Geometry: final body of the model. Coordinates: model frame, mm. A direction names the side the tool comes from. Round coordinates to 2 decimals unless told otherwise and drop trailing zeros. Order: outer loops, then holes, each group sorted by start corner. A loop starts at its lowest first (then second) coordinate and runs counter-clockwise, first axis right, second up. Notation, with made-up numbers: (-23, 78) - (5, 78) arc R11 cw to (5, 99) - close; hole circle Ø11 at (-5.5, 59.5). An arc over 180 degrees is marked (long way). Put each result on its own line as item: value. Start each with the question number.
(1) Pin query (flat end, axial travel): P1, Ø1, axis at x = 344, z = -137, coming from the +Y side; P2, Ø8, axis at x = -549, z = -4.5, coming from the +Y side; P3, Ø4, axis at y = 0, z = -1803.4, coming from the +X side; P4, Ø1, axis at x = 394.5, y = -102.5, coming from the -Z side. Return the tip coordinate at first contact, or that it passes through.
(2) Access query for faces 1 (the face through (-1, 25.4, -1465)), 2 (the face through (-510.54, -7, -229)), 3 (the face through (684.768, -8.392, -284.552)), 4 (the face through (345.44, -7, -42)), 5 (the face through (-586.74, -7, -228)). Directions: +Z, -Z, +X, -X, +Y, -Y. A direction counts if a zero-diameter tool reaches every point of the face in a straight line with its end or side. Return the directions, or none.
(3) Material intervals for L1, parallel to Z at x = -7.5, y = 0; L2, parallel to Z at x = 6.5, y = 0; L3, parallel to Z at x = 579, y = 201.5, sorted ascending. Write a range as [from, to].
(4) Section D-D (z = -1072.5). Output: boundary loops of the cut face in (x, y).
(5) Section C-C (y = 374). Output: boundary loops of the cut face in (x, z), and give its area (3 significant figures).
(6) Section B-B (x = 0). Output: boundary loops of the cut face in (y, z) (1 decimal).
(7) Section A-A (x = 420). Output: boundary loops of the cut face in (y, z), and give its area (3 significant figures).
(8) Pull-direction query (X, two-part tool) for faces 6 (the face through (-345.44, -7, -48)), 7 (the face through (-2, 36, -1397)), 8 (the face through (242.165, -2.134, -1326.863)), 9 (the face through (-50.8, -1, -996)); classes: released by +X, released by -X, zero draft, split by the parting line, or undercut.
from build123d import *

# Parameters (mm, degrees)
F1_DEPTH      = 599.44
F2_W          = 127
F2_H          = 457.2
F2_R          = 1.5875
F3_DEPTH      = 751.841
F3_DEPTH_BACK = 751.841


with BuildPart() as f1:
    # F0 (on Front) → F1 (new body, symmetric)
    with BuildSketch(Plane.XZ):
        with BuildLine():
            Line((751.84, 203.2), (345.44, 203.2))
            Line((345.44, 203.2), (345.44, -203.2))
            Line((345.44, -203.2), (510.54, -203.2))
            Line((510.54, -203.2), (510.54, -254))
            Line((510.54, -254), (0, -254))
            Line((0, -254), (-510.54, -254))
            Line((-510.54, -254), (-510.54, -203.2))
            Line((-510.54, -203.2), (-345.44, -203.2))
            Line((-345.44, -203.2), (-345.44, 203.2))
            Line((-345.44, 203.2), (-751.84, 203.2))
            Line((-751.84, 203.2), (-751.84, -203.2))
            Line((-751.84, -203.2), (-586.74, -203.2))
            Line((-586.74, -203.2), (-586.74, -254))
            Line((-586.74, -254), (-612.14, -254))
            ThreePointArc((-612.14, -254), (-683.9820489686, -283.7579510314), (-713.74, -355.6))
            Line((-713.74, -355.6), (-713.74, -726.44))
            ThreePointArc((-713.74, -726.44), (-683.9820489686, -798.2820489686), (-612.14, -828.04))
            Line((-612.14, -828.04), (-50.8, -828.04))
            Line((-50.8, -828.04), (-50.8, -1168.4))
            Line((-50.8, -1168.4), (-200.6969981396, -1168.4))
            ThreePointArc((-200.6969981396, -1168.4), (-266.3715614854, -1205.9568669833), (-267.3077825801, -1281.6059913558))
            Line((-267.3077825801, -1281.6059913558), (-217.7162994978, -1370.8706609039))
            ThreePointArc((-217.7162994978, -1370.8706609039), (-199.0711985486, -1389.9830422305), (-173.3091098709, -1397))
            Line((-173.3091098709, -1397), (-50.8, -1397))
            Line((-50.8, -1397), (-50.8, -1534.8474755722))
            ThreePointArc((-50.8, -1534.8474755722), (-151.8342242526, -1691.6513427765), (-25.4, -1828.8))
            Line((-25.4, -1828.8), (25.4, -1828.8))
            ThreePointArc((25.4, -1828.8), (151.8342242526, -1691.6513427765), (50.8, -1534.8474755722))
            Line((50.8, -1534.8474755722), (50.8, -1397))
            Line((50.8, -1397), (173.3091098709, -1397))
            ThreePointArc((173.3091098709, -1397), (199.0711985486, -1389.9830422305), (217.7162994978, -1370.8706609039))
            Line((217.7162994978, -1370.8706609039), (267.3077825801, -1281.6059913558))
            ThreePointArc((267.3077825801, -1281.6059913558), (266.3715614854, -1205.9568669833), (200.6969981396, -1168.4))
            Line((200.6969981396, -1168.4), (50.8, -1168.4))
            Line((50.8, -1168.4), (50.8, -828.04))
            Line((50.8, -828.04), (612.14, -828.04))
            ThreePointArc((612.14, -828.04), (683.9820489686, -798.2820489686), (713.74, -726.44))
            Line((713.74, -726.44), (713.74, -355.6))
            ThreePointArc((713.74, -355.6), (683.9820489686, -283.7579510314), (612.14, -254))
            Line((612.14, -254), (586.74, -254))
            Line((586.74, -254), (586.74, -203.2))
            Line((586.74, -203.2), (751.84, -203.2))
            Line((751.84, -203.2), (751.84, 203.2))
        make_face()
        with BuildLine():
            ThreePointArc((0, -1589.6315735093), (88.9, -1678.5315735093), (0, -1767.4315735093))
            ThreePointArc((0, -1767.4315735093), (-88.9, -1678.5315735093), (0, -1589.6315735093))
        make_face(mode=Mode.SUBTRACT)
    extrude(amount=F1_DEPTH, both=True)

    # F2 (on Right) → F3 (cut, two sides)
    with BuildSketch(Plane.YZ) as f3_sk:
        with Locations((535.94, -25.4)):
            Rectangle(F2_W, F2_H)
        Polygon((599.44, -1828.8), (599.44, -828.04), (152.4, -828.04), (76.2, -828.04), (76.2, -1168.4), (152.4, -1168.4), (152.4, -1397), (25.4, -1397), (25.4, -1534.8474755722), (38.1, -1534.8474755722), (38.1, -1828.8), align=None)
        Polygon((203.2, 0), (38.1, 0), (38.1, 203.2), (0, 203.2), (-38.1, 203.2), (-38.1, 0), (-203.2, 0), (-203.2, -38.1), (0, -38.1), (203.2, -38.1), align=None)
        Polygon((-76.2, -828.04), (-152.4, -828.04), (-599.44, -828.04), (-599.44, -1828.8), (-38.1, -1828.8), (-38.1, -1534.8474755722), (-25.4, -1534.8474755722), (-25.4, -1397), (-152.4, -1397), (-152.4, -1168.4), (-76.2, -1168.4), align=None)
        with Locations((-535.94, -25.4)):
            Rectangle(F2_W, F2_H)
        with Locations((0, -1803.4)):
            Circle(F2_R)
    extrude(amount=-F3_DEPTH, mode=Mode.SUBTRACT)
    extrude(f3_sk.sketch, amount=F3_DEPTH_BACK, mode=Mode.SUBTRACT)


solid = f1.part
Checks:
1. P1: passes through
1. P2: stops at y = 472.44
1. P3: stops at x = 90.16
1. P4: stops at z = -828.04
2. face 1: +X, -X, +Y
2. face 2: +Y, -Y
2. face 3: +X, +Y, -Y
2. face 4: +Z, +Y, -Y
2. face 5: -X, +Y, -Y
3. L1: z = [-1828.8, -1804.99], [-1801.81, -1767.11], [-1589.95, -254]
3. L2: z = [-1828.8, -1804.99], [-1801.81, -1767.19], [-1589.87, -254]
3. L3: z = [-828.04, -38.1], [0, 203.2]
4. outline: (-50.8, -76.2) - (50.8, -76.2) - (50.8, 76.2) - (-50.8, 76.2) - close
5. outline: (-751.84, -203.2) - (-586.74, -203.2) - (-586.74, -254) - (-612.14, -254) arc R101.6 ccw to (-713.74, -355.6) - (-713.74, -726.44) arc R101.6 ccw to (-612.14, -828.04) - (612.14, -828.04) arc R101.6 ccw to (713.74, -726.44) - (713.74, -355.6) arc R101.6 ccw to (612.14, -254) - (586.74, -254) - (586.74, -203.2) - (751.84, -203.2) - (751.84, 203.2) - (345.44, 203.2) - (345.44, -203.2) - (510.54, -203.2) - (510.54, -254) - (-510.54, -254) - (-510.54, -203.2) - (-345.44, -203.2) - (-345.44, 203.2) - (-751.84, 203.2) - close
5. area: 1,150,000 mm²
6. outline: (-599.4, -828) - (-76.2, -828) - (-76.2, -1168.4) - (-152.4, -1168.4) - (-152.4, -1397) - (-25.4, -1397) - (-25.4, -1534.8) - (-38.1, -1534.8) - (-38.1, -1589.6) - (38.1, -1589.6) - (38.1, -1534.8) - (25.4, -1534.8) - (25.4, -1397) - (152.4, -1397) - (152.4, -1168.4) - (76.2, -1168.4) - (76.2, -828) - (599.4, -828) - (599.4, -254) - (-599.4, -254) - close; (-38.1, -1828.8) - (38.1, -1828.8) - (38.1, -1767.4) - (-38.1, -1767.4) - close; hole circle Ø3.2 at (0, -1803.4)
7. outline: (-599.44, -828.04) - (599.44, -828.04) - (599.44, -254) - (-599.44, -254) - close; (-472.44, -203.2) - (472.44, -203.2) - (472.44, 203.2) - (38.1, 203.2) - (38.1, 0) - (203.2, 0) - (203.2, -38.1) - (-203.2, -38.1) - (-203.2, 0) - (-38.1, 0) - (-38.1, 203.2) - (-472.44, 203.2) - close
7. area: 1,040,000 mm²
8. face 6: undercut
8. face 7: zero draft
8. face 8: released by +X
8. face 9: released by -X
